Can you work these out from the model? Positions are in its coordinate system, mm. Give positions to 0.01 mm unless a question says otherwise; leave off trailing zeros. Order: outer loops, then holes, each group sorted by start corner. A loop starts at its lowest first (then second) coordinate and runs counter-clockwise, first axis right, second up. Notation, with made-up numbers: (2, -35.75) - (12, -35.75) arc R38 ccw to (12, 3.25) - close; hole circle Ø1 at (14, 55). An arc over 180 degrees is marked (long way). Answer as CSV lines item,"result".
```python
from build123d import *

# Parameters (mm, degrees)
F1_DEPTH = 2.54
F2_R     = 0.508
F3_DEPTH = 25.4
F4_R     = 0.508


with BuildPart() as f1:
    # F0 (on Front) → F1 (new body)
    with BuildSketch(Plane.XZ):
        Polygon((-10.16, 2.54), (-10.16, 0), (-10.16, -2.54), (-7.112, -4.299764), (-7.112, -8.89), (3.048, -8.89), (3.048, -4.299764), (0, -2.54), (0, 0), (0, 2.54), (3.048, 4.299764), (3.048, 8.89), (-7.112, 8.89), (-7.112, 4.299764), align=None)
    extrude(amount=F1_DEPTH)

    # F2 (on face) → F3 (cut)
    with BuildSketch(Plane.XY.offset(8.89)):
        with Locations((1.524, -1.27)):
            Circle(F2_R)
        with Locations((-8.7376, -1.27)):
            Circle(F2_R)
    extrude(amount=-F3_DEPTH, mode=Mode.SUBTRACT)

    # F4
    f4_edges = [f1.edges().sort_by_distance(p)[0] for p in [
        (-10.16, 0, 0),
        (-8.636, 0, -3.419882),
        (-7.112, 0, -6.594882),
        (-2.032, 0, -8.89),
        (3.048, 0, -6.594882),
        (1.524, 0, -3.419882),
        (0, 0, 0),
        (1.524, 0, 3.419882),
        (3.048, 0, 6.594882),
        (-2.032, 0, 8.89),
        (-7.112, 0, 6.594882),
        (-8.636, 0, 3.419882),
        (-10.16, -2.54, 0),
        (-8.636, -2.54, -3.419882),
        (-7.112, -2.54, -6.594882),
        (-2.032, -2.54, -8.89),
        (3.048, -2.54, -6.594882),
        (1.524, -2.54, -3.419882),
        (0, -2.54, 0),
        (1.524, -2.54, 3.419882),
        (3.048, -2.54, 6.594882),
        (-2.032, -2.54, 8.89),
        (-7.112, -2.54, 6.594882),
        (-8.636, -2.54, 3.419882),
        (3.048, -1.27, -8.89),
        (-7.112, -1.27, 8.89),
        (-7.112, -1.27, 4.299764),
        (-10.16, -1.27, 2.54),
        (3.048, -1.27, 8.89),
        (3.048, -1.27, -4.299764),
        (3.048, -1.27, 4.299764),
        (0, -1.27, 2.54),
        (0, -1.27, -2.54),
        (-7.112, -1.27, -8.89),
        (-7.112, -1.27, -4.299764),
        (-10.16, -1.27, -2.54),
    ]]
    fillet(f4_edges, radius=F4_R)


solid = f1.part
```
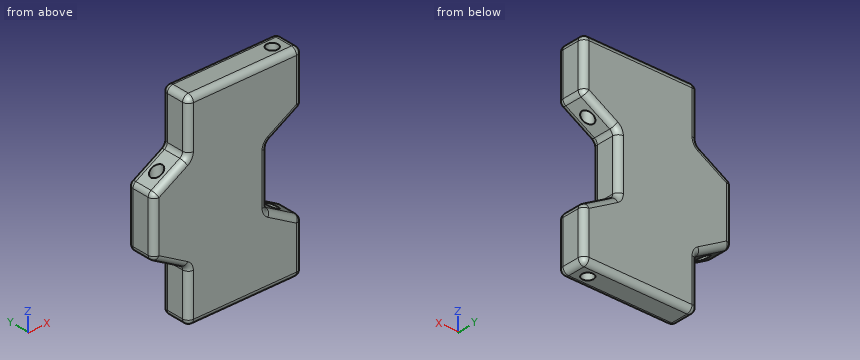
1) I want a section at B-B on y = -0.2. Write out the boundary of the cut face in (x, z), plus the area to 3 significant figures.
Answer block:
outline,"(-10.06, -2.25) arc R0.4 ccw to (-9.85, -2.6) - (-7.31, -4.06) arc R0.61 cw to (-7.01, -4.59) - (-7.01, -8.38) arc R0.4 ccw to (-6.6, -8.79) - (2.54, -8.79) arc R0.4 ccw to (2.94, -8.38) - (2.94, -4.59) arc R0.4 ccw to (2.74, -4.24) - (0.2, -2.78) arc R0.61 cw to (-0.1, -2.25) - (-0.1, 2.25) arc R0.61 cw to (0.2, 2.78) - (2.74, 4.24) arc R0.4 ccw to (2.94, 4.59) - (2.94, 8.38) arc R0.4 ccw to (2.54, 8.79) - (-6.6, 8.79) arc R0.4 ccw to (-7.01, 8.38) - (-7.01, 4.59) arc R0.61 cw to (-7.31, 4.06) - (-9.85, 2.6) arc R0.4 ccw to (-10.06, 2.25) - close"
area,"174 mm2"
2) I'm going to push flat-ended pins straight in: P1, Ø0.5, axis at y = -1.5, z = 7, coming from the -X side; P2, Ø0.8, axis at y = -1, z = 0.5, coming from the +X side; P3, Ø1.3, axis at x = -8.74, y = -1.27, coming from the -Z side. Where does each tip first touch, or does it pass through?
Answer block:
P1,"x = -7.11"
P2,"x = 0"
P3,"z = -3.74"
3) I need wall thicknesses on line 1 along X through (y, z) = (-1.27, 6.4); line 2 along X through (y, z) = (-0.6, -5.75); line 3 along X through (y, z) = (-1.6, 7.75). Which ranges of each line are inside material? Lowest first, please. Write a range as [from, to].
Answer block:
line 1,"[-7.11, 1.02], [2.03, 3.05]"
line 2,"[-7.11, 3.05]"
line 3,"[-7.11, 1.14], [1.91, 3.05]"
4) I want a section at C-C on y = -1.27. Count the separate pieces of the cut face and the enclosed holes in it, plus the area to 3 significant figures.
Answer block:
separate pieces,"4"
enclosed holes,"0"
area,"162 mm2"
5) I want a section at A-A on z = 1.25. Write out the boundary of the cut face in (x, y), plus the area to 3 significant figures.
Answer block:
outline,"(-10.16, -2.03) arc R0.51 ccw to (-9.65, -2.54) - (-0.51, -2.54) arc R0.51 ccw to (0, -2.03) - (0, -0.51) arc R0.51 ccw to (-0.51, 0) - (-9.65, 0) arc R0.51 ccw to (-10.16, -0.51) - close; hole circle Ø1.02 at (-8.74, -1.27)"
area,"24.8 mm2"
